Geometry: final body of the model. Coordinates: model frame, mm. A direction names the side the tool comes from. Coordinates: 2 decimals unless noted, no trailing zeros. Order: outer loops, then holes, each group sorted by start corner. A loop starts at its lowest first (then second) coordinate and runs counter-clockwise, first axis right, second up. Notation, with made-up numbers: M -28,-22 L 23,-22 A13 ccw 23,-8 Z; hole C 57,-27 d8. An arc over 180 degrees is marked long. Use CSV: the item, a comma, the result in double quotes. Start each with the question number.
Q1. Mould query, pull axis X, two halves, no side actions, for faces 4 (the face through (-4.4, -8.5, 0.3)), 5 (the face through (5, -19, 0)), 6 (the face through (0.35, -17.79, 6.44)), 7 (the face through (23.846, -4.934, 7.509)). Classes: +X half, -X half, draft (parallel to the pull), parting line (faces both ways), or undercut.
Q2. Section query C-C, the plane y = -1.5. Output: boundary loops of the cut face in (x, z), and give its area (3 significant figures).
Q3. Section query B-B, the plane x = 9. State how many separate pieces and enclosed holes the cut face has, and give its area (3 significant figures).
Q4. Section query A-A, the plane y = -11. Output: boundary loops of the cut face in (x, z).
Q5. First-contact query: P1, Ø10, axis at x = -14.5, y = -4, coming from the +Z side; P2, Ø21, axis at x = 5.5, z = 5, coming from the +Y side; P3, Ø8, axis at y = -13.5, z = -13, coming from the -X side. Flat tips, straight axial feed; report the tip coordinate or a pass-through.
Q6. Access query for faces 1 (the face through (-20.03, -4.19, 6.31)), 2 (the face through (11.923, -17.99, 3.755)), 3 (the face through (6, -13.5, -2.5)). Directions: +Z, -Z, +X, -X, +Y, -Y. A direction counts if a zero-diameter tool reaches every point of the face in a straight line with its end or side. Return the directions, or none.
Q7. Ray query, probe 1 along Y at (x, z) = (-4.5, 6); probe 2 along Z at (x, y) = (0, -16.9); probe 3 along X at (y, z) = (-6.5, 0.5) (3 decimals). Return the intervals inside material, ascending.
from build123d import *

# Parameters (mm, degrees)
F0_R      = 25
F1_DEPTH  = 10
F2_R      = 6.5
F3_DEPTH  = 7
F4_R      = 12.5
F5_DEPTH  = 2
F6_R      = 4
F7_DEPTH  = 19.001
F9_D      = 3.2
F9_DEPTH  = 4.25
F9_TIP    = 0.9613769904
F10_R     = 0.3
F11_R     = 21
F11_R_2   = 4
F12_DEPTH = 8.5


with BuildPart() as f1:
    # F0 (on Front) → F1 (new body)
    with BuildSketch(Plane.XZ):
        Circle(F0_R)
    extrude(amount=F1_DEPTH)

    # F2 (on face) → F3 (join)
    with BuildSketch(Plane.XZ.offset(10)):
        Circle(F2_R)
    extrude(amount=F3_DEPTH)

    # F4 (on face) → F5 (join)
    with BuildSketch(Plane.XZ.offset(17)):
        Circle(F4_R)
    extrude(amount=F5_DEPTH)

    # F6 (on face) → F7 (cut, through all)
    with BuildSketch(Plane.XZ.offset(19)):
        Circle(F6_R)
    extrude(amount=-F7_DEPTH, mode=Mode.SUBTRACT)

    # F9
    with Locations(Plane.XZ.offset(19)):
        with Locations((-8, 0), (0, 8), (8, 0), (0, -8)):
            Hole(F9_D / 2, depth=F9_DEPTH)
            with Locations((0, 0, -(F9_DEPTH + F9_TIP / 2))):  # 118° drill point
                Cone(0, F9_D / 2, F9_TIP, mode=Mode.SUBTRACT)

    # F10
    f10_edges = [f1.edges().sort_by_distance(p)[0] for p in [
        (-25, -10, 0),
        (-25, 0, 0),
        (-12.5, -19, 0),
        (-12.5, -17, 0),
        (-4, -19, 0),
    ]]
    fillet(f10_edges, radius=F10_R)

    # F11 (on face) → F12 (cut)
    with BuildSketch(Plane(origin=(0, 0, 0), x_dir=(-1, 0, 0), z_dir=(0, 1, 0))):
        Circle(F11_R)
        Circle(F11_R_2, mode=Mode.SUBTRACT)
    extrude(amount=-F12_DEPTH, mode=Mode.SUBTRACT)


solid = f1.part
Responses:
1,face 4,"undercut"
1,face 5,"draft"
1,face 6,"undercut"
1,face 7,"parting line"
2,outline,"C 0,0 d50; hole C 0,0 d42"
2,area,"578 mm²"
3,separate pieces,"3"
3,enclosed holes,"0"
3,area,"173 mm²"
4,outline,"C 0,0 d13; hole C 0,0 d8"
5,P1,"stops at z = 23.12"
5,P2,"stops at y = -8.5"
5,P3,"stops at x = -22.24"
6,face 1,"+Y"
6,face 2,"-Y"
6,face 3,"none"
7,probe 1,"y = -19 to -17, -10 to -8.5"
7,probe 2,"z = -6.4 to -4, 4 to 6.4"
7,probe 3,"x = -24.995 to -20.994, 20.994 to 24.995"
